Here's how the part is built. I have some questions about the finished solid (model axes, mm). Face numbers are marked on the shaded views. A direction names the side the tool comes from. Coordinates: 2 decimals unless noted, no trailing zeros. Write each loop counter-clockwise with the first axis right and the second up, starting at its lowest first coordinate (ties: lowest second). Pieces come first, ordered by that corner, then holes. Notation, with made-up numbers: (76.5, 65.5) -> (91.5, 65.5) arc R28 cw to (91.5, 88.5) -> close; hole circle Ø8 at (49.5, 10). An arc over 180 degrees is marked (long way). Answer in a Markdown table with one row per item. Add a question column.
from build123d import *

# Parameters (mm, degrees)
F2_DEPTH = 10


with BuildPart() as f2:
    # F1 (on Top) → F2 (new body)
    with BuildSketch(Plane.XY):
        Polygon((-23.7262713233, -0.5133114427), (-29.9929815414, -0.6488900181), (-18.8932398178, -14.3612300563), (-16.6224315579, -12.6351311898), (-1.9995321028, -0.0432593345), (-20.8745733923, -0.4516157317), align=None)
        Polygon((-24.646239762, 17.1044691702), (-23.7262713233, -0.5133114427), (-20.8745733923, -0.4516157317), (-1.6430826508, 1.1402979447), (-17.1533376915, 11.904401586), (-19.4966736096, 13.5306746951), align=None)
        Polygon((-9.8854720883, 28.324502495), (-19.4966736096, 13.5306746951), (-17.1533376915, 11.904401586), (-0.6590314726, 1.8883001663), (-6.8801100131, 19.7133421136), (-7.8200092446, 22.4064029902), align=None)
        Polygon((8.6512099282, 28.7255385812), (-7.8200092446, 22.4064029902), (-6.8801100131, 19.7133421136), (0.5767473285, 1.9150359054), (6.021085844, 19.9924559857), (6.8436328595, 22.7236469086), align=None)
        Polygon((23.883423796, 18.1543952744), (6.8436328595, 22.7236469086), (6.021085844, 19.9924559857), (1.5922282531, 1.2102930183), (16.6224315579, 12.6351311898), (18.8932398178, 14.3612300563), align=None)
        Polygon((20.8745733923, 0.4516157317), (23.7262713233, 0.5133114427), (29.9929815414, 0.6488900181), (18.8932398178, 14.3612300563), (16.6224315579, 12.6351311898), (1.9995321028, 0.0432593345), align=None)
        Polygon((17.1533376915, -11.904401586), (19.4966736096, -13.5306746951), (24.646239762, -17.1044691702), (23.7262713233, 0.5133114427), (20.8745733923, 0.4516157317), (1.6430826508, -1.1402979447), align=None)
        Polygon((6.8801100131, -19.7133421136), (7.8200092446, -22.4064029902), (9.8854720883, -28.324502495), (19.4966736096, -13.5306746951), (17.1533376915, -11.904401586), (0.6590314726, -1.8883001663), align=None)
        Polygon((-6.021085844, -19.9924559857), (-6.8436328595, -22.7236469086), (-8.6512099282, -28.7255385812), (7.8200092446, -22.4064029902), (6.8801100131, -19.7133421136), (-0.5767473285, -1.9150359054), align=None)
        Polygon((-16.6224315579, -12.6351311898), (-18.8932398178, -14.3612300563), (-23.883423796, -18.1543952744), (-6.8436328595, -22.7236469086), (-6.021085844, -19.9924559857), (-1.5922282531, -1.2102930183), align=None)
    extrude(amount=F2_DEPTH)


solid = f2.part
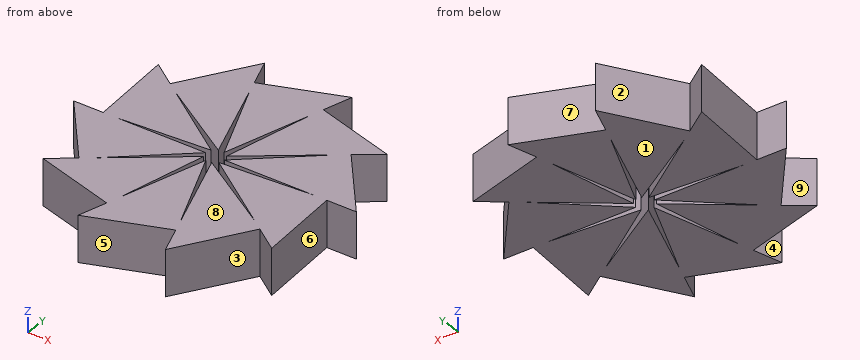
Q1. I need wall thicknesses on line 1 (X direction, y = 15, z = 5); line 2 (X direction, y = 4, z = 4); line 3 (X direction, y = 9, z = 3.25). Which ranges of each line are inside material? Lowest first, please. Write a range as [from, to].
Q2. Imagine slicing it at D-D on y = 8.5. Please give me the cut outline in (x, z).
Q3. Imagine slicing it at B-B on x = 13. Please give me the cut outline in (y, z), plus the area to 3 significant figures.
Q4. I'm going to push flat-ended pins straight in: P1, Ø1, axis at x = -10.5, y = 7.5, coming from the +Z side; P2, Ø1, axis at y = -0.5, z = 4, coming from the +X side; P3, Ø1.5, axis at x = -6.5, z = 7.5, coming from the -Y side; P4, Ø2, axis at y = -12.5, z = 3.5, coming from the -X side. Where does each tip first touch, or does it pass through?
Q5. For the marked faces 5, 6, 7, 8 and 9, which set-ups out of +Z, -Z, +X, -X, +Y, -Y let a thin tool reach every point of the face, with its end or its side?
Q6. Imagine slicing it at A-A on y = 16. Please give me the cut outline in (x, z), plus the area to 3 significant figures.
Q7. If we mould it in two halves opening along Y, with no side actions, what happens to the marked faces 1, 2, 3 and 4? For each: pulls with the +Y half, pulls with the -Y half, needs draft (parallel to the pull), parting line crosses it, or undercut.
Q8. Imagine slicing it at C-C on y = -4. Please give me the cut outline in (x, z), plus the area to 3 significant figures.
Result sheet:
| question | item | result |
|---|---|---|
| 1 | line 1 | x = [-24.54, -21.61], [-18.54, -5.24], [-4.91, 4.52], [4.84, 19.73] |
| 1 | line 2 | x = [-23.96, -5.76], [-4.14, -1.4], [-0.3, 1.2], [2.25, 5.26], [6.59, 27.28] |
| 1 | line 3 | x = [-24.22, -12.97], [-12.37, -3.14], [-2.39, 2.71], [3.43, 11.84], [12.4, 23.23] |
| 2 | outline | (-24.2, 0) -> (-12.25, 0) -> (-12.25, 10) -> (-24.2, 10) -> close; (-11.55, 0) -> (-2.97, 0) -> (-2.97, 10) -> (-11.55, 10) -> close; (-2.18, 0) -> (2.56, 0) -> (2.56, 10) -> (-2.18, 10) -> close; (3.31, 0) -> (11.18, 0) -> (11.18, 10) -> (3.31, 10) -> close; (11.82, 0) -> (23.64, 0) -> (23.64, 10) -> (11.82, 10) -> close |
| 3 | outline | (-23.53, 0) -> (-9.38, 0) -> (-9.38, 10) -> (-23.53, 10) -> close; (-9.02, 0) -> (-0.2, 0) -> (-0.2, 10) -> (-9.02, 10) -> close; (0.28, 0) -> (9.52, 0) -> (9.52, 10) -> (0.28, 10) -> close; (9.88, 0) -> (21.07, 0) -> (21.07, 10) -> (9.88, 10) -> close |
| 3 | area | 434 mm^2 |
| 4 | P1 | stops at z = 10 |
| 4 | P2 | stops at x = 23.81 |
| 4 | P3 | stops at y = -28.19 |
| 4 | P4 | stops at x = -21.21 |
| 5 | face 5 | +Z, -Z, -Y |
| 5 | face 6 | +Z, -Z, +X |
| 5 | face 7 | +Z, -Z, +Y |
| 5 | face 8 | +Z, +X, -X, +Y, -Y |
| 5 | face 9 | +Z, -Z, -X |
| 6 | outline | (-24.59, 0) -> (-23.05, 0) -> (-23.05, 10) -> (-24.59, 10) -> close; (-17.89, 0) -> (-5.58, 0) -> (-5.58, 10) -> (-17.89, 10) -> close; (-5.32, 0) -> (4.82, 0) -> (4.82, 10) -> (-5.32, 10) -> close; (5.08, 0) -> (21.05, 0) -> (21.05, 10) -> (5.08, 10) -> close |
| 6 | area | 400 mm^2 |
| 7 | face 1 | needs draft |
| 7 | face 2 | pulls with the +Y half |
| 7 | face 3 | pulls with the -Y half |
| 7 | face 4 | undercut |
| 8 | outline | (-27.28, 0) -> (-6.59, 0) -> (-6.59, 10) -> (-27.28, 10) -> close; (-5.26, 0) -> (-2.25, 0) -> (-2.25, 10) -> (-5.26, 10) -> close; (-1.2, 0) -> (0.3, 0) -> (0.3, 10) -> (-1.2, 10) -> close; (1.4, 0) -> (4.14, 0) -> (4.14, 10) -> (1.4, 10) -> close; (5.76, 0) -> (23.96, 0) -> (23.96, 10) -> (5.76, 10) -> close |
| 8 | area | 461 mm^2 |
